Build history of the part. All positions in model axes, mm. Round coordinates to 2 decimals unless told otherwise and drop trailing zeros. Write each loop counter-clockwise with the first axis right and the second up, starting at its lowest first coordinate (ties: lowest second). Pieces come first, ordered by that corner, then holes.
1) Wall check: probe 1 along Z at (x, y) = (19, 121); probe 2 along X at (y, z) = (284.5, -26). Give the ranges that are in metal, low to high.
2) Saw through at B-B (z = -25.5). Write the cut outline in (x, y), plus the area to 3 significant figures.
3) Saw through at A-A (x = 22). Write the cut outline in (y, z).
4) Saw through at C-C (y = 289). Write the cut outline in (x, z).
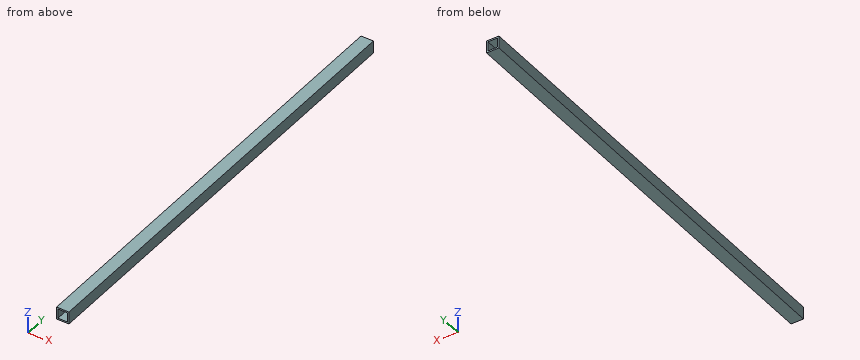
from build123d import *

# Parameters (mm, degrees)
SKETCH1_W           = 8.5
SKETCH1_H           = 8.5
SKETCH1_W_2         = 6.5
SKETCH1_H_2         = 6.5
BOSS_EXTRUDE1_DEPTH = 310


with BuildPart() as part:
    # Sketch1 → Boss-Extrude1 (new body)
    with BuildSketch(Plane(origin=(0, 0, 0), x_dir=(1, 0, 0), z_dir=(0, 1, 0))):
        with Locations((20.126704545, 26.085227273)):
            Rectangle(SKETCH1_W, SKETCH1_H)
        with Locations((20.126704545, 26.085227273)):
            Rectangle(SKETCH1_W_2, SKETCH1_H_2, mode=Mode.SUBTRACT)
    extrude(amount=BOSS_EXTRUDE1_DEPTH)


solid = part.part
Evaluation:
1. probe 1: z = -30.34 to -29.34, -22.84 to -21.84
1. probe 2: x = 15.88 to 16.88, 23.38 to 24.38
2. outline: (15.88, 0) - (16.88, 0) - (16.88, 310) - (15.88, 310) - close; (23.38, 0) - (24.38, 0) - (24.38, 310) - (23.38, 310) - close
2. area: 620 mm2
3. outline: (0, -30.34) - (310, -30.34) - (310, -29.34) - (0, -29.34) - close; (0, -22.84) - (310, -22.84) - (310, -21.84) - (0, -21.84) - close
4. outline: (15.88, -30.34) - (24.38, -30.34) - (24.38, -21.84) - (15.88, -21.84) - close; hole (16.88, -29.34) - (23.38, -29.34) - (23.38, -22.84) - (16.88, -22.84) - close
